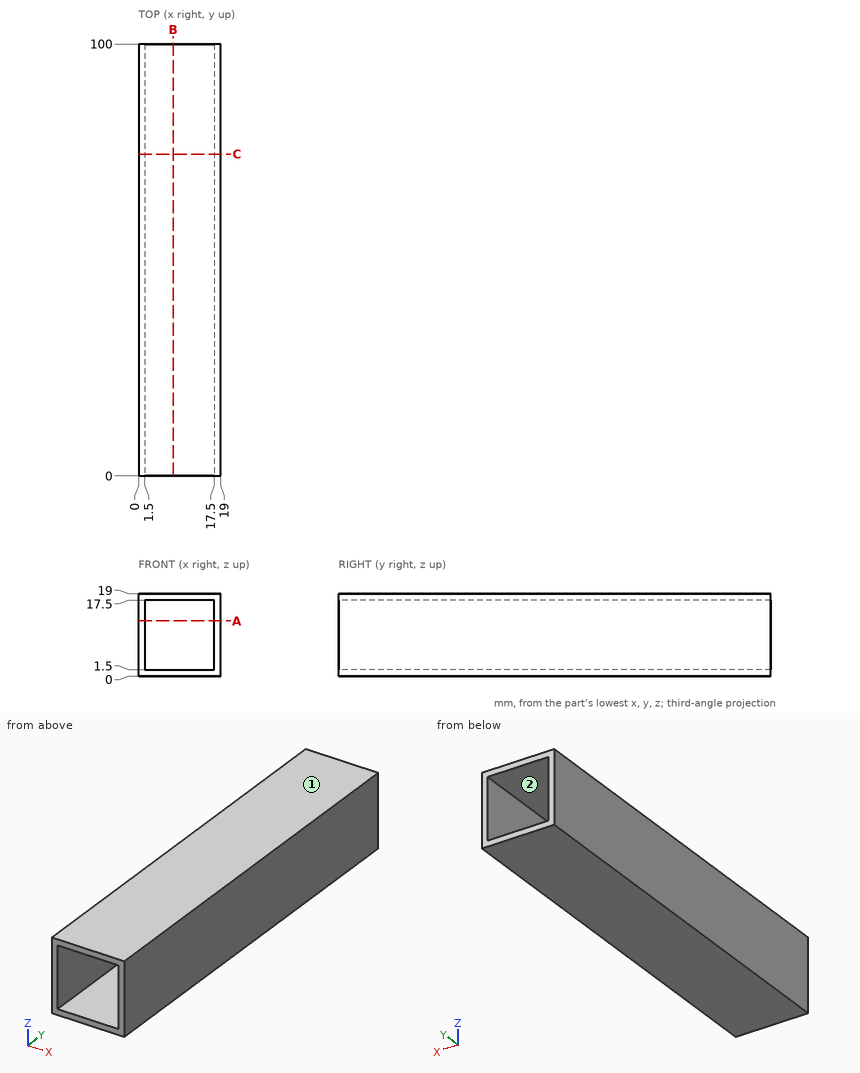
The drawing under review shows one solid part. Ordinate dimensions are in mm from its lowest x, y, z. A direction names the side the tool comes from. Coordinates: 2 decimals unless noted, no trailing zeros. Write each loop counter-clockwise with the first axis right and the second up, starting at its lowest first coordinate (ties: lowest second). Pieces come first, ordered by that corner, then holes.
1) Add section A-A (z = 12.75). Write out the cut boundary in (x, y), plus the area to 3 significant figures.
2) Add section B-B (x = 8). Write out the cut boundary in (y, z).
3) To check wall thickness, follow L1, parallel to Z at x = 16, y = 70. State the ranges of the line that lie inside material, in increasing order.
4) Machinability: for the marked faces 1 and 2, which of the approach directions +Z, -Z, +X, -X, +Y, -Y give a long, thin tool a straight path to every point of the face, cutting with its end or side? Answer none if there is none.
5) Insertion check: pin 1 (3 mm diameter, centred on x = 15, z = 13, fed in from +Y). The pin has a flat end and moves straight along its axis. Give the tip position at first contact, or say it passes through.
6) Add section C-C (y = 74.5). Write out the cut boundary in (x, z).
Check result:
1. outline: (0, 0) - (1.5, 0) - (1.5, 100) - (0, 100) - close; (17.5, 0) - (19, 0) - (19, 100) - (17.5, 100) - close
1. area: 300 mm2
2. outline: (0, 0) - (100, 0) - (100, 1.5) - (0, 1.5) - close; (0, 17.5) - (100, 17.5) - (100, 19) - (0, 19) - close
3. L1: z = 0 to 1.5, 17.5 to 19
4. face 1: +Z, +X, -X, +Y, -Y
4. face 2: +Y, -Y
5. pin 1: passes through
6. outline: (0, 0) - (19, 0) - (19, 19) - (0, 19) - close; hole (1.5, 1.5) - (17.5, 1.5) - (17.5, 17.5) - (1.5, 17.5) - close
